For this review, take the finished solid that the model builds, in its own axes (mm). A direction names the side the tool comes from. Coordinates: 2 decimals unless noted, no trailing zeros. Write each loop counter-clockwise with the first axis right and the second up, starting at its lowest first coordinate (ties: lowest second). Pieces come first, ordered by that corner, then holes. Notation, with made-up numbers: M 29.5,60.5 L 84.5,60.5 A14 cw 84.5,71.5 Z; hole C 33,-1.75 d7. An arc over 180 degrees is marked long. One line per question, with ' | ' between items.
from build123d import *

# Parameters (mm, degrees)
SKETCH1_W           = 164
SKETCH1_H           = 164
BOSS_EXTRUDE1_DEPTH = 5
BOSS_EXTRUDE2_DEPTH = 5
SKETCH3_R           = 3.5
SKETCH3_R_2         = 2.5
BOSS_EXTRUDE3_DEPTH = 5
SKETCH5_W           = 125.8
SKETCH5_H           = 129.9
CUT_EXTRUDE1_DEPTH  = 117.073252733
CHAMFER2_SIZE       = 10
BOSS_EXTRUDE4_DEPTH = 20
SKETCH7_W           = 3.272727273
SKETCH7_H           = 1.402597403
SKETCH7_W_2         = 1.636363636
SKETCH7_H_2         = 9
CUT_EXTRUDE3_DEPTH  = 1.5


with BuildPart() as part:
    # Sketch1 → Boss-Extrude1 (new body)
    with BuildSketch(Plane(origin=(0, 0, 0), x_dir=(1, 0, 0), z_dir=(0, 1, 0))):
        Rectangle(SKETCH1_W, SKETCH1_H)
    extrude(amount=BOSS_EXTRUDE1_DEPTH)

    # Sketch2 → Boss-Extrude2 (add)
    with BuildSketch(Plane(origin=(0, 5, 0), x_dir=(1, 0, 0), z_dir=(0, 1, 0))):
        Polygon((-80, -80), (-80, 82), (-82, 82), (-82, -82), (82, -82), (82, 82), (80, 82), (80, -80), (24.75, -80), (24.75, -74.9), (74.9, -74.9), (74.9, 82), (72.9, 82), (72.9, -72.9), (-72.9, -72.9), (-72.9, 82), (-74.9, 82), (-74.9, -74.9), (-24.75, -74.9), (-24.75, -80), align=None)
    extrude(amount=BOSS_EXTRUDE2_DEPTH)

    # Sketch3 → Boss-Extrude3 (add)
    with BuildSketch(Plane(origin=(0, 5, 0), x_dir=(1, 0, 0), z_dir=(0, 1, 0))):
        with Locations(Location((-24.75, -67.9, 0), (0, 0, 270))):
            Circle(SKETCH3_R)
        with Locations(Location((-24.75, -67.9, 0), (0, 0, 270))):
            Circle(SKETCH3_R_2, mode=Mode.SUBTRACT)
    extrude(amount=BOSS_EXTRUDE3_DEPTH)

    # Sketch5 → Cut-Extrude1 (cut, through all)
    with BuildSketch(Plane(origin=(0, 5, 0), x_dir=(1, 0, 0), z_dir=(0, 1, 0))):
        with Locations((0, 7.05)):
            Rectangle(SKETCH5_W, SKETCH5_H)
    extrude(amount=-CUT_EXTRUDE1_DEPTH, mode=Mode.SUBTRACT)

    # Chamfer2
    # the kernel refuses this chamfer: 10 mm, written as the material it adds along each edge
    with BuildSketch(Plane(origin=(98.61682988, 5, 72.9), x_dir=(0, -0.027495876610586403, -0.9996219169112968), z_dir=(-1, 0, 0))) as chamfer2_piece_1_section:
        Polygon((CHAMFER2_SIZE * 0.999621916911, -CHAMFER2_SIZE * 0.0274958766106), (-CHAMFER2_SIZE * 0.0274958766106, -CHAMFER2_SIZE * 0.999621916911), (0, 0), align=None)
    chamfer2_piece_1 = extrude(amount=171.51682988, mode=Mode.PRIVATE)
    chamfer2_piece_1 = split(chamfer2_piece_1, bisect_by=Plane(origin=(0.76457013, 10, 69.034324166), z_dir=(0, -1, 0)), keep=Keep.TOP, mode=Mode.PRIVATE)
    chamfer2_piece_1 = split(chamfer2_piece_1, bisect_by=Plane(origin=(74.9, 7.221559046, 69.034324166), z_dir=(-1, 0, 0)), keep=Keep.TOP, mode=Mode.PRIVATE)
    chamfer2_piece_1 = chamfer2_piece_1 - Plane(origin=(-24.75, 7.221559046, 67.9), x_dir=(0, 0, 1), z_dir=(0, -1, 0)) * Cylinder(2.5, 384, mode=Mode.PRIVATE)
    add(chamfer2_piece_1)

    # Sketch6 → Boss-Extrude4 (add, symmetric)
    with BuildSketch(Plane(origin=(0, 0, 0), x_dir=(0, 0, -1), z_dir=(1, 0, 0))):
        Polygon((-82, 0), (-82, 10), (-102, 1.5), (-102, 0), align=None)
    extrude(amount=BOSS_EXTRUDE4_DEPTH, both=True)

    # Sketch7 → Cut-Extrude3 (cut)
    # profile 1 of 4: a face of its own
    with BuildSketch(Plane(origin=(0, -16.938205466, 145.38401286), x_dir=(1, 0, 0), z_dir=(0, -0.9203309184584746, -0.39114064034485163))):
        Polygon((-8.649350649, -60.736982492), (-8.649350649, -58.633086388), (-5.961038961, -58.633086388), (-5.961038961, -57.230488986), (-8.649350649, -57.230488986), (-8.649350649, -54.542177297), (-4.675324675, -54.542177297), (-4.675324675, -53.139579895), (-10.285714286, -53.139579895), (-10.285714286, -62.139579895), (-4.675324675, -62.139579895), (-4.675324675, -60.736982492), align=None)
    # profile 2 of 4: a face of its own
    with BuildSketch(Plane(origin=(0, -16.938205466, 145.38401286), x_dir=(1, 0, 0), z_dir=(0, -0.9203309184584746, -0.39114064034485163))):
        with Locations((-1.753246754, -56.762956519)):
            Rectangle(SKETCH7_W, SKETCH7_H)
    # profile 3 of 4: a face of its own
    with BuildSketch(Plane(origin=(0, -16.938205466, 145.38401286), x_dir=(1, 0, 0), z_dir=(0, -0.9203309184584746, -0.39114064034485163))):
        Polygon((6.779220779, -53.139579895), (6.118100649, -55.009709765), (2.978693182, -55.009709765), (2.337662338, -53.139579895), (0.584415584, -53.139579895), (4.207792208, -62.256463012), (4.909090909, -62.256463012), (8.532467532, -53.139579895), align=None)
        Polygon((4.558441558, -59.568151323), (3.444399351, -56.295424051), (5.648741883, -56.295424051), align=None, mode=Mode.SUBTRACT)
    # profile 4 of 4: a face of its own
    with BuildSketch(Plane(origin=(0, -16.938205466, 145.38401286), x_dir=(1, 0, 0), z_dir=(0, -0.9203309184584746, -0.39114064034485163))):
        with Locations((10.285714286, -57.639579895)):
            Rectangle(SKETCH7_W_2, SKETCH7_H_2)
    extrude(amount=CUT_EXTRUDE3_DEPTH, mode=Mode.SUBTRACT)


solid = part.part
1) Machinability: for faces 4 (the flat face through (-1, 3, -72)), 5 (the flat face through (20, 3, 90)), 6 (the flat face through (6.695, 4.974, 91.935)), which of the approach directions +Z, -Z, +X, -X, +Y, -Y give a long, thin tool a straight path to every point of the face, cutting with its end or side? Answer none if there is none.
Responses:
face 4: +Y, -Y | face 5: +Z, +X, +Y, -Y | face 6: none
2) The part is to be moulded in two halves that separate along Z. For faces 1 (the flat face through (53, 7, 80)), 2 (the flat face through (-51, 5, 82)), 3 (the flat face through (72.9, 7, -8)), say which applies: +Z half, -Z half, draft (parallel to the pull), parting line (faces both ways), or undercut.
Responses:
face 1: undercut | face 2: +Z half | face 3: draft
3) We need section A-A on z = 17. State the section outline as (x, y) points, then the cut area to 3 significant figures.
Responses:
outline: M -82,0 L -62.9,0 L -62.9,5 L -72.9,5 L -72.9,10 L -74.9,10 L -74.9,5 L -80,5 L -80,10 L -82,10 Z; M 62.9,0 L 82,0 L 82,10 L 80,10 L 80,5 L 74.9,5 L 74.9,10 L 72.9,10 L 72.9,5 L 62.9,5 Z | area: 231 mm^2
4) Insertion check: pin 1 Ø3 at (y, z) = (7, 95) entering from +X; pin 2 Ø1.2 at (y, z) = (4, 93.5) entering from -X; pin 3 Ø2.5 at (y, z) = (4.5, 91.5) entering from +X; pin 4 Ø2.5 at (x, y) = (-44, 8.5) entering from +Z. Each pin has a flat end and moves straight along its axis. Give the tip position at first contact, or say it passes through.
Responses:
pin 1: through | pin 2: x = -20 | pin 3: x = 20 | pin 4: z = 82
5) We need section B-B on x = -59. State the section outline as (y, z) points, then the cut area to 3 significant figures.
Responses:
outline: M 0,-82 L 5,-82 L 5,-72 L 0,-72 Z; M 0,57.9 L 5,57.9 L 5,62.9 L 10,67.9 L 10,74.9 L 5,74.9 L 5,80 L 10,80 L 10,82 L 0,82 Z | area: 228 mm^2
6) To check wall thickness, follow line 1 along X through (y, z) = (7, -50); line 2 along X through (y, z) = (6.85, 67.9); line 3 along Z through (x, y) = (-47.5, 7.5). State the ranges of each line that lie inside material, in increasing order. Write a range as [from, to].
Responses:
line 1: [-82, -80], [-74.9, -72.9], [72.9, 74.9], [80, 82] | line 2: [-82, -80], [-74.9, -27.25], [-22.25, 74.9], [80, 82] | line 3: [65.4, 74.9], [80, 82]
